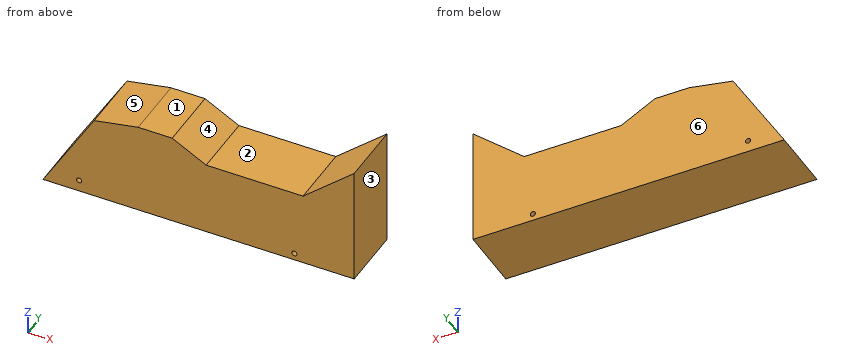
```python
from build123d import *

# Parameters (mm, degrees)
F0_R     = 1.075
F1_DEPTH = 26.6
F2_DEPTH = 158
F4_DEPTH = 26.601


# Not quite as in the source:
# - an extrude ends at something that could not be found from the text; its depth is read off the source's solid


with BuildPart() as f1:
    # F0 (on Front) → F1 (new body)
    with BuildSketch(Plane.XZ):
        Polygon((50, 25), (-50, 25), (-80, -25), (-50, -25), (25, -25), (50, -25), align=None)
        with Locations((-64.9039745331, -20)):
            Circle(F0_R, mode=Mode.SUBTRACT)
        with Locations((25, -22)):
            Circle(F0_R, mode=Mode.SUBTRACT)
    extrude(amount=F1_DEPTH)

    # F0 (on Front) → F2 (cut, through all)
    with BuildSketch(Plane.XZ):
        with Locations((-64.9039745331, -20)):
            Circle(F0_R)
    extrude(amount=-F2_DEPTH, mode=Mode.SUBTRACT)

    # F3 (on face) → F4 (cut, through all)
    with BuildSketch(Plane(origin=(0, 0, 0), x_dir=(-1, 0, 0), z_dir=(0, 1, 0))):
        Polygon((50, 25), (-50, 25), (-28.6072827876, 6.4954175614), (11.8362475187, 6.4954175614), (26.036022231, 14.1141144559), (40.2304567397, 14.1141144559), (58.63198501, 10.6133583166), align=None)
    extrude(amount=-F4_DEPTH, mode=Mode.SUBTRACT)


solid = f1.part
```
For this review, take the finished solid that the model builds, in its own axes (mm). Face numbers are marked on the shaded views. A direction names the side the tool comes from. Give positions to 0.01 mm unless a question says otherwise; leave off trailing zeros. Order: outer loops, then holes, each group sorted by start corner. A loop starts at its lowest first (then second) coordinate and runs counter-clockwise, first axis right, second up.
1) Insertion check: pin 1 (3 mm diameter, centred on x = -22.5, y = -18.5, fed in from +Z); pin 2 (7 mm diameter, centred on x = -31.5, y = -18, fed in from +Z); pin 3 (12 mm diameter, centred on y = -13, z = -1, fed in from -X). Each pin has a flat end and moves straight along its axis. Give the tip position at first contact, or say it passes through.
2) The part is to be moulded in two halves that separate along X. For the marked faces 4, 5 and 6, say which applies: released by +X, released by -X, zero draft, split by the parting line, or undercut.
3) Wall thickness on line 1 (Z direction, x = 25, y = -9.25) (3 decimals); line 2 (Z direction, x = 7.5, y = -0.75); line 3 (Z direction, x = -64.5, y = -12): over which ranges is each line inside the solid? List them lowest first.
4) For the marked faces 1, 2 and 3, list the 3-axis set-ups (+Z, -Z, +X, -X, +Y, -Y) from which the entire face can be reached by the end or side of a thin tool; tool diameter is ignored.
5) Take a section at C-C (x = 31). Give the boundary of the cut face in (y, z).
6) Take a section at A-A (y = -24.25). Give the boundary of the cut face in (x, z) (3 decimals).
7) Take a section at B-B (z = 3). Give the boundary of the cut face in (x, y).
Derived:
1. pin 1: stops at z = 13.02
1. pin 2: stops at z = 14.11
1. pin 3: stops at x = -69.2
2. face 4: undercut
2. face 5: released by -X
2. face 6: zero draft
3. line 1: z = -25 to -23.075, -20.925 to 6.495
3. line 2: z = -25 to 6.5
3. line 3: z = -25 to -21, -19 to 0.83
4. face 1: +Z, -X, +Y, -Y
4. face 2: +Z, +Y, -Y
4. face 3: +Z, -Z, +X, +Y, -Y
5. outline: (-26.6, -25) - (0, -25) - (0, 8.57) - (-26.6, 8.57) - close
6. outline: (-80, -25) - (50, -25) - (50, 25) - (28.607, 6.495) - (-11.836, 6.495) - (-26.036, 14.114) - (-40.23, 14.114) - (-58.632, 10.613) - close; hole circle Ø2.15 at (-64.904, -20); hole circle Ø2.15 at (25, -22)
7. outline: (-63.2, -26.6) - (50, -26.6) - (50, 0) - (-63.2, 0) - close
